Here's the drawing with two shaded views (mm, measured from the low corner). I have some questions. A direction names the side the tool comes from. Give positions to 0.01 mm unless a question says otherwise; leave off trailing zeros. Loops run counter-clockwise (first coordinate to the right, second up) from the corner with the lowest first, then second, coordinate; pieces in that order, holes last. Notation, with made-up numbers: M 34.5,-13 L 48.5,-13 A25 ccw 48.5,1 Z; hole C 85.25,80.5 d6. An arc over 180 degrees is marked long. Use a Markdown table: item, result. Add a question column.
1) Suppose I cut it at D-D on x = 11.5. List the corners of the cut face in (y, z) for me, and give its area (3 significant figures).
2) Suppose I cut it at A-A on x = 5.75. List the corners of the cut face in (y, z) for me.
3) Which directions (+Z, -Z, +X, -X, +Y, -Y) give clear straight access to the entire face, cutting with the end or side of a thin tool? Please do the marked faces 4, 5, 6, 7 and 8.
4) We'd pull the mould along Z, two halves only. Please class the marked faces 1, 2 and 3: +Z half, -Z half, draft (parallel to the pull), parting line (faces both ways), or undercut.
5) Suppose I cut it at C-C on y = 13.25. List the corners of the cut face in (x, z) for me.
6) Will these pins go through, and if not, where does the flat tip stop? pin 1 Ø1 at (x, y) = (7.5, 7.5) entering from -Z; pin 2 Ø2 at (x, z) = (3, 6) entering from +Y; pin 3 Ø2.5 at (x, y) = (16, 5) entering from -Z.
7) If I drill on line 1 along X through (y, z) = (19, 10.5); line 2 along Z through (x, y) = (15.25, 20.5); line 3 along X through (y, z) = (4.5, 11), over which ranges is the centre line in solid material (lowest first)? Write a range as [from, to].
8) Suppose I cut it at B-B on z = 10.25. List the corners of the cut face in (x, y) for me, and give its area (3 significant figures).
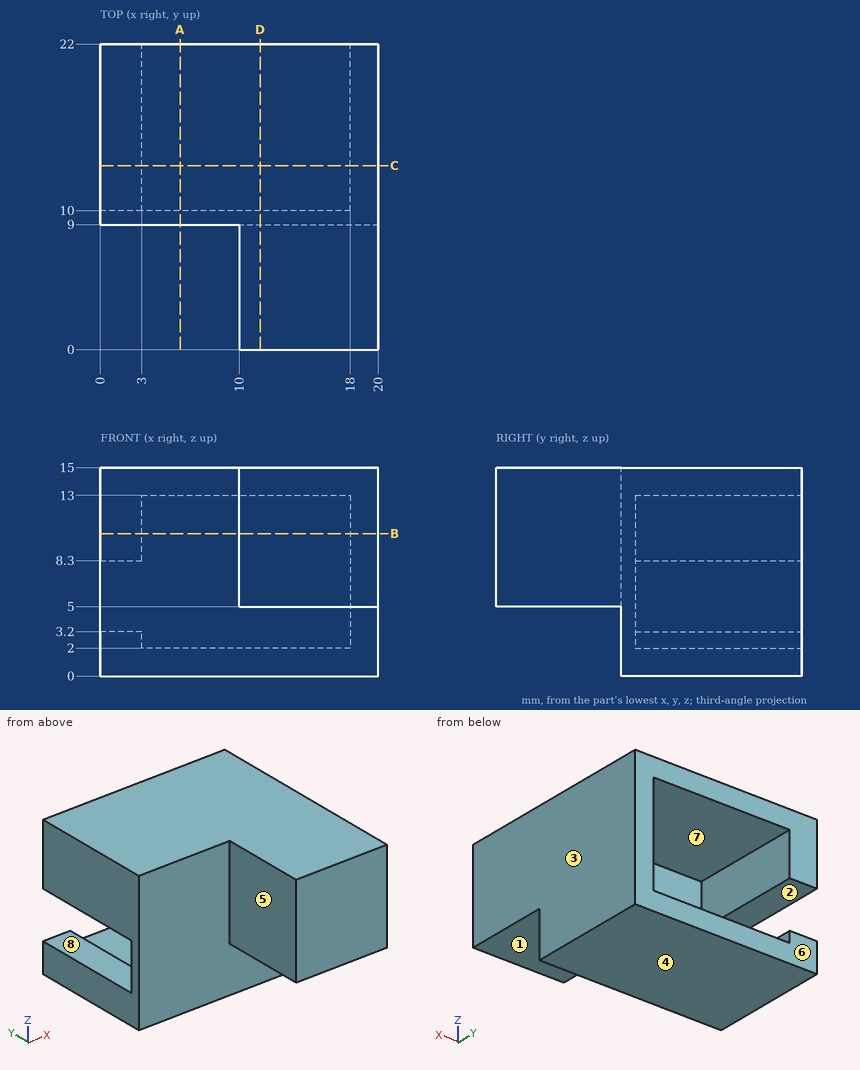
Answer block:
| question | item | result |
|---|---|---|
| 1 | outline | M 0,5 L 9,5 L 9,0 L 22,0 L 22,2 L 10,2 L 10,13 L 22,13 L 22,15 L 0,15 Z |
| 1 | area | 153 mm^2 |
| 2 | outline | M 9,0 L 22,0 L 22,2 L 10,2 L 10,13 L 22,13 L 22,15 L 9,15 Z |
| 3 | face 4 | -Z, +X, -X, +Y, -Y |
| 3 | face 5 | +Z, -Z, -X, -Y |
| 3 | face 6 | +Z, -Z, +X, -X, +Y |
| 3 | face 7 | +Y |
| 3 | face 8 | -X, +Y |
| 4 | face 1 | -Z half |
| 4 | face 2 | undercut |
| 4 | face 3 | draft |
| 5 | outline | M 0,0 L 20,0 L 20,15 L 0,15 L 0,8.3 L 3,8.3 L 3,13 L 18,13 L 18,2 L 3,2 L 3,3.2 L 0,3.2 Z |
| 6 | pin 1 | passes through |
| 6 | pin 2 | stops at y = 10 |
| 6 | pin 3 | stops at z = 5 |
| 7 | line 1 | x = [0, 3], [18, 20] |
| 7 | line 2 | z = [0, 2], [13, 15] |
| 7 | line 3 | x = [10, 20] |
| 8 | outline | M 0,9 L 10,9 L 10,0 L 20,0 L 20,22 L 18,22 L 18,10 L 3,10 L 3,22 L 0,22 Z |
| 8 | area | 170 mm^2 |
